```python
from build123d import *

# Parameters (mm, degrees)
F0_R     = 63.5
F0_R_2   = 20.32
F1_DEPTH = 12.7
F0_R_3   = 12.7
F2_DEPTH = 76.2
F3_W     = 127
F3_H     = 12.7
F4_DEPTH = 6.35


with BuildPart() as f1:
    # F0 (on Top) → F1 (new body)
    with BuildSketch(Plane.XY):
        Circle(F0_R)
        Circle(F0_R_2, mode=Mode.SUBTRACT)
    extrude(amount=F1_DEPTH)

    # F0 (on Top) → F2 (join)
    with BuildSketch(Plane.XY):
        Circle(F0_R_2)
        Circle(F0_R_3, mode=Mode.SUBTRACT)
    extrude(amount=F2_DEPTH)

    # F3 (on Top) → F4 (cut)
    with BuildSketch(Plane.XY):
        with Locations((-63.5, 0)):
            Rectangle(F3_W, F3_H)
    extrude(amount=F4_DEPTH, mode=Mode.SUBTRACT)


solid = f1.part
```
Design review of the part built by this model. Coordinates are the model's own, in mm. A direction names the side the tool comes from. Coordinates: 2 decimals unless noted, no trailing zeros. Loops run counter-clockwise (first coordinate to the right, second up) from the corner with the lowest first, then second, coordinate; pieces in that order, holes last.
Q1. We need section A-A on x = 0. State the section outline as (y, z) points, and give its area (3 significant figures).
Reported:
outline: (-63.5, 0) - (-12.7, 0) - (-12.7, 76.2) - (-20.32, 76.2) - (-20.32, 12.7) - (-63.5, 12.7) - close; (12.7, 0) - (63.5, 0) - (63.5, 12.7) - (20.32, 12.7) - (20.32, 76.2) - (12.7, 76.2) - close
area: 2,260 mm2
Q2. The part is to be moulded in two halves that separate along X. For faces 1 (the face through (13, 1, 0)), 2 (the face through (12.114, 3.815, 37.567)), 3 (the face through (60.57, 19.07, 6.26)), say which applies: +X half, -X half, draft (parallel to the pull), parting line (faces both ways), or undercut.
Reported:
face 1: draft
face 2: undercut
face 3: parting line
Q3. For pin 1 (3 mm diameter, centred on x = -22.5, z = 25, fed in from -Y); pin 2 (1.9 mm diameter, centred on x = -31, z = 4.5, fed in from -Y); pin 3 (3 mm diameter, centred on x = 2.5, z = 9.5, fed in from -Y); pin 4 (1.5 mm diameter, centred on y = -6, z = 45, fed in from +X), all flat-tipped, find the tip position at first contact; note any pin that passes through.
Reported:
pin 1: passes through
pin 2: stops at y = -55.94
pin 3: stops at y = -63.49
pin 4: stops at x = 19.63
Q4. To check wall thickness, follow line 1 (Y direction, x = 0, z = 50); line 2 (Z direction, x = -19, y = 4); line 3 (Z direction, x = 20, y = 34). State the ranges of each line that lie inside material, in increasing order.
Reported:
line 1: y = -20.32 to -12.7, 12.7 to 20.32
line 2: z = 6.35 to 76.2
line 3: z = 0 to 12.7
Q5. Tool access review of faces 4 (the face through (-37, -6.35, 3)), 5 (the face through (0, -13, 76.2)), 6 (the face through (-2.645, 20.147, 44.006)): name each direction out of +Z, -Z, +X, -X, +Y, -Y from which nothing blocks a thin tool from reaching the whole face with its end or side.
Reported:
face 4: -Z, -X
face 5: +Z, +X, -X, +Y, -Y
face 6: +Z
Q6. We need section B-B on y = 0. State the section outline as (x, z) points, and give its area (3 significant figures).
Reported:
outline: (-63.5, 6.35) - (-12.7, 6.35) - (-12.7, 76.2) - (-20.32, 76.2) - (-20.32, 12.7) - (-63.5, 12.7) - close; (12.7, 0) - (63.5, 0) - (63.5, 12.7) - (20.32, 12.7) - (20.32, 76.2) - (12.7, 76.2) - close
area: 1,940 mm2
Q7. We need section D-D on x = -36. State the section outline as (y, z) points.
Reported:
outline: (-52.31, 0) - (-6.35, 0) - (-6.35, 6.35) - (6.35, 6.35) - (6.35, 0) - (52.31, 0) - (52.31, 12.7) - (-52.31, 12.7) - close
Q8. We need section C-C on z = 41. State the section outline as (x, y) points, and give its area (3 significant figures).
Reported:
outline: circle Ø40.64 at (0, 0); hole circle Ø25.4 at (0, 0)
area: 790 mm2
